Solid Edge part; units mm, degrees
sketch "Sketch1" plane through (0, 0, 0) normal (0, 0, 1) x (1, 0, 0)
  circle A0 centre (0, 0) radius 5
extrude "Protrusion1" add sketch "Sketch1" along normal mid plane 10
chamfer "Chamfer1" distance 0.75 angle 45 2 edges at (-5, 0, -5) (-5, 0, 5)
sketch "Sketch2" plane through (0, 0, 5) normal (0, 0, 1) x (1, 0, 0)
  line L0 (-1.4434, 2.5) -> (1.4434, 2.5)
  line L1 (2.8868, 0) -> (1.4434, 2.5)
  line L2 (1.4434, -2.5) -> (2.8868, 0)
  line L3 (-1.4434, -2.5) -> (1.4434, -2.5)
  line L4 (-2.8868, 0) -> (-1.4434, -2.5)
  line L5 (-1.4434, 2.5) -> (-2.8868, 0)
extrude "Cutout1" cut sketch "Sketch2" against normal blind 5
properties part number "24104460"
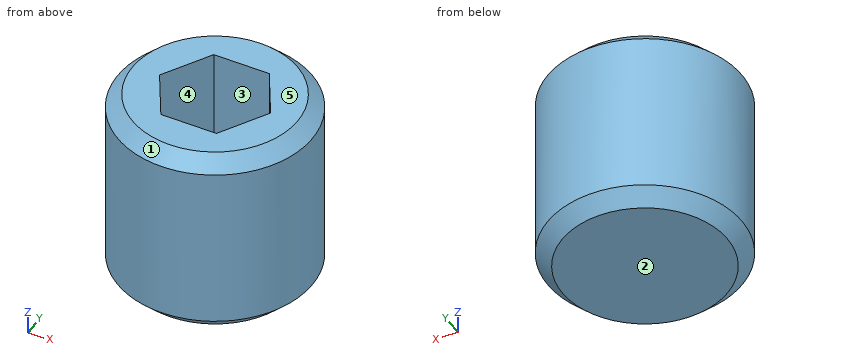
Source: CAD feature listing. Evaluate the final solid. Frame: model axes, mm. Face numbers are marked on the shaded views. A direction names the side the tool comes from. Give positions to 0.01 mm unless a question says otherwise; leave off trailing zeros. Order: outer loops, then holes, each group sorted by start corner. A loop starts at its lowest first (then second) coordinate and runs counter-clockwise, first axis right, second up.
(1) Section query A-A (z = 2). Return the cut outline in (x, y), plus the area to 3 significant figures.
(2) Pull-direction query (Y, two-part tool) for the marked faces 1, 2 and 3; classes: +Y half, -Y half, draft (parallel to the pull), parting line (faces both ways), or undercut.
(3) Contact query for flat-ended pins moving along their axis: P1, Ø1.5, axis at x = 1.5, y = 0, coming from the +Z side; P2, Ø1, axis at y = -3, z = 0.5, coming from the +X side; P3, Ø1.5, axis at x = 2.5, z = 3, coming from the -Y side. Output: stop coordinate, or through.
(4) Section query C-C (z = -3.5). Return the cut outline in (x, y), plus the area to 3 significant figures.
(5) Material intervals for line 1 along Z through (x, y) = (-1, 0); line 2 along Y through (x, z) = (-2.5, 3.5); line 3 along Y through (x, z) = (0.5, -1.25), sorted ascending.
(6) Section query B-B (x = 0). Return the cut outline in (y, z), plus the area to 3 significant figures.
(7) Access query for the marked faces 4 and 5. Directions: +Z, -Z, +X, -X, +Y, -Y. A direction counts if a zero-diameter tool reaches every point of the face in a straight line with its end or side. Return the directions, or none.
Outcome:
1. outline: circle Ø10 at (0, 0); hole (-2.89, 0) - (-1.44, -2.5) - (1.44, -2.5) - (2.89, 0) - (1.44, 2.5) - (-1.44, 2.5) - close
1. area: 56.9 mm2
2. face 1: parting line
2. face 2: draft
2. face 3: undercut
3. P1: stops at z = 0
3. P2: stops at x = 4.33
3. P3: stops at y = -4.68
4. outline: circle Ø10 at (0, 0)
4. area: 78.5 mm2
5. line 1: z = -5 to 0
5. line 2: y = -4.33 to -0.67, 0.67 to 4.33
5. line 3: y = -4.97 to 4.97
6. outline: (-5, -4.25) - (-4.25, -5) - (4.25, -5) - (5, -4.25) - (5, 4.25) - (4.25, 5) - (2.5, 5) - (2.5, 0) - (-2.5, 0) - (-2.5, 5) - (-4.25, 5) - (-5, 4.25) - close
6. area: 73.9 mm2
7. face 4: +Z
7. face 5: +Z, +X, -X, +Y, -Y
